Model file for the job. Use its own axes, mm. A direction names the side the tool comes from. Coordinates: 2 decimals unless noted, no trailing zeros. Write each loop counter-clockwise with the first axis right and the second up, starting at its lowest first coordinate (ties: lowest second). Pieces come first, ordered by that corner, then holes. Notation, with made-up numbers: M 51.5,74 L 69.5,74 A8 cw 69.5,88 Z; hole C -12.75,12.5 d3. An arc over 180 degrees is marked long. Answer in a Markdown table with one row per item. Add a question column.
```python
from build123d import *

# Parameters (mm, degrees)
SKETCH_W        = 126
SKETCH_H        = 25
SKETCH_R        = 2.2
PAD_DEPTH       = 3
SKETCH001_W     = 12.4
SKETCH001_H     = 4
PAD001_DEPTH    = 21.497
SKETCH002_R     = 2.2
POCKET_DEPTH    = 4
CHAMFER_SIZE    = 1
FILLET_R        = 1.5
SKETCH003_W     = 41.75
SKETCH003_H     = 9.7
SKETCH003_W_2   = 16.2
SKETCH003_H_2   = 13.6
POCKET001_DEPTH = 24.498
SKETCH004_W     = 2.651
SKETCH004_H     = 0.381966
POCKET002_DEPTH = 15.808


with BuildPart() as part:
    # Sketch → Pad (new body)
    with BuildSketch(Plane.XY):
        Rectangle(SKETCH_W, SKETCH_H)
        with Locations((-53, 0.726)):
            Circle(SKETCH_R, mode=Mode.SUBTRACT)
        with Locations((53, 0.726)):
            Circle(SKETCH_R, mode=Mode.SUBTRACT)
    extrude(amount=PAD_DEPTH)

    # Sketch001 → Pad001 (new body)
    with BuildSketch(Plane.XY.offset(3)):
        with Locations((-38.154, -3.892)):
            Rectangle(SKETCH001_W, SKETCH001_H)
        with Locations((38.154, -3.892)):
            Rectangle(SKETCH001_W, SKETCH001_H)
    extrude(amount=PAD001_DEPTH)

    # Sketch002 → Pocket (cut)
    with BuildSketch(Plane.XZ.offset(5.892)):
        with Locations((-38.154, 18.297)):
            Circle(SKETCH002_R)
    pocket = extrude(amount=-POCKET_DEPTH, mode=Mode.SUBTRACT)

    # Mirrored: Pocket across Sketch002 V_Axis
    add(pocket.mirror(Plane(origin=(0, -5.892, 0), x_dir=(0, -1, 0), z_dir=(1, 0, 0))), mode=Mode.SUBTRACT)

    # Chamfer
    chamfer_edges = [part.edges().sort_by_distance(p)[0] for p in [
        (0, 12.5, 0),
        (63, 0, 0),
        (0, -12.5, 0),
        (-63, 0, 0),
        (50.8, 0.726, 0),
        (-55.2, 0.726, 0),
    ]]
    chamfer(chamfer_edges, length=CHAMFER_SIZE)

    # Fillet
    fillet_edges = [part.edges().sort_by_distance(p)[0] for p in [
        (38.154, -5.892, 3),
        (31.954, -3.892, 3),
        (38.154, -1.892, 3),
        (44.354, -3.892, 3),
        (-38.154, -5.892, 3),
        (-31.954, -3.892, 3),
        (-38.154, -1.892, 3),
        (-44.354, -3.892, 3),
    ]]
    fillet(fillet_edges, radius=FILLET_R)

    # Sketch003 → Pocket001 (cut, through all)
    with BuildSketch(Plane(origin=(0, 0, 0), x_dir=(1, 0, 0), z_dir=(0, 0, -1))):
        with Locations((-12.23, 1.542)):
            Rectangle(SKETCH003_W, SKETCH003_H)
        with Locations((21.425, -0.408)):
            Rectangle(SKETCH003_W_2, SKETCH003_H_2)
    extrude(amount=-POCKET001_DEPTH, mode=Mode.SUBTRACT)

    # Sketch004 → Pocket002 (cut)
    with BuildSketch(Plane.XZ.offset(12.5)):
        with Locations((-31.7795, 3.190983)):
            Rectangle(SKETCH004_W, SKETCH004_H)
    extrude(amount=-POCKET002_DEPTH, mode=Mode.SUBTRACT)


solid = part.part
```
1) Two-plate mould, pull along X, no slides. Class faces 1 (the face through (38, -4, 24.497)), 2 (the face through (-55.2, 0.8, 2)), 3 (the face through (44.354, -4, 14)): released by +X, released by -X, zero draft, split by the parting line, or undercut.
2) Slice it at A-A (x = -5). Give the cut face in (y, z), then the cut area to 3 significant figures.
3) Drill centre lines: probe 1 along Y at (x, z) = (-53, 2.1); probe 2 along Y at (x, z) = (-26.5, 2.25); probe 3 along Z at (x, y) = (10, 0). Where is each one in solid material? Low to high.
4) Slice it at C-C (y = -8.5). Give the cut face in (x, z), then the cut area to 3 significant figures.
5) Slice it at D-D (x = -53). Give the cut face in (y, z).
6) Slice it at B-B (z = 5.75). Give the cut face in (x, y) (3 decimals), then the cut area to 3 significant figures.
7) Flat gauge pins, fed straight in: pin 1 Ø5.5 at (x, y) = (53, 0.726) entering from +Z; pin 2 Ø3.5 at (x, z) = (39.5, 18.5) entering from +Y; pin 3 Ø12 at (y, z) = (-7.5, 16.5) entering from +X. Where does each tip first touch, or does it go through?
8) Which spindle directions (+Z, -Z, +X, -X, +Y, -Y) get a long thin tool onto all of the face, cutting with end or side? Do faces 4 (the face through (-39, -1.892, 14)), 5 (the face through (31.954, -4, 14)), 6 (the face through (38, -5.892, 14)), 7 (the face through (29.525, 1, 1)). Say none if no direction does.
Ans:
| question | item | result |
|---|---|---|
| 1 | face 1 | zero draft |
| 1 | face 2 | undercut |
| 1 | face 3 | released by +X |
| 2 | outline | M -12.5,1 L -11.5,0 L -6.39,0 L -6.39,3 L -12.5,3 Z; M 3.31,0 L 11.5,0 L 12.5,1 L 12.5,3 L 3.31,3 Z |
| 2 | area | 44.9 mm2 |
| 3 | probe 1 | y = -12.5 to -1.47, 2.93 to 12.5 |
| 3 | probe 2 | y = -12.5 to -6.39, 3.31 to 12.5 |
| 3 | probe 3 | z = 0 to 3 |
| 4 | outline | M -63,1 L -62,0 L 62,0 L 63,1 L 63,3 L -63,3 Z |
| 4 | area | 377 mm2 |
| 5 | outline | M -12.5,1 L -11.5,0 L -2.47,0 L -1.47,1 L -1.47,3 L -12.5,3 Z; M 2.93,1 L 3.93,0 L 11.5,0 L 12.5,1 L 12.5,3 L 2.93,3 Z |
| 6 | outline | M -44.354,-5.892 L -33.105,-5.892 L -33.105,-1.892 L -44.354,-1.892 Z; M 31.954,-5.892 L 44.354,-5.892 L 44.354,-1.892 L 31.954,-1.892 Z |
| 6 | area | 94.6 mm2 |
| 7 | pin 1 | stops at z = 3 |
| 7 | pin 2 | stops at y = -1.89 |
| 7 | pin 3 | stops at x = 44.35 |
| 8 | face 4 | +Z, +X, -X, +Y |
| 8 | face 5 | +Z, +Y, -Y |
| 8 | face 6 | +Z, +X, -X, -Y |
| 8 | face 7 | +Z, -Z |
